Geometry check sheet. Reference: the model listing, model coordinates, mm. Face numbers are marked on the shaded views. A direction names the side the tool comes from. Give positions to 0.01 mm unless a question says otherwise; leave off trailing zeros. Loops run counter-clockwise (first coordinate to the right, second up) from the corner with the lowest first, then second, coordinate; pieces in that order, holes last. Notation, with made-up numbers: (-37.75, 47.5) -> (-33.75, 47.5) arc R13 ccw to (-33.75, 52.5) -> close; hole circle Ø3 at (38, 17). An arc over 180 degrees is marked (long way). Answer in a Markdown table with one row per item. Add a question column.
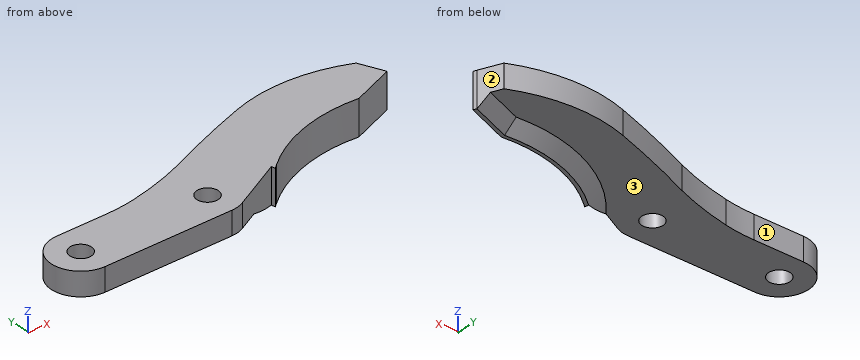
Autodesk Inventor part; units mm, degrees
ref_plane "YZ Plane" through (0, 0, 0) normal (1, 0, 0) x (0, 1, 0)
ref_plane "XZ Plane" through (0, 0, 0) normal (0, 1, 0) x (-1, 0, 0)
ref_plane "XY Plane" through (0, 0, 0) normal (0, 0, 1) x (1, 0, 0)
sketch "Náčrt1" plane through (0, 0, 0) normal (0, 0, 1) x (1, 0, 0)
  circle A0 centre (0, 0) radius 1.825
  circle A1 centre (22, 0) radius 1.825
  arc A2 (0, 5) -> (0, -5) centre (0, 0) ccw
  line L0 (0, 0) -> (-0.516, 0)
  line L1 (0, 5) -> (8.645, 5)
  arc A3 (8.645, 5) -> (13.8862, 5.4744) centre (8.645, 34.19) ccw
  arc A4 (8.645, 5) -> (8.645, 5) centre (6.8603, 48.5893) ccw
  arc A5 (58.5138, 12.7037) -> (38.8579, 13.8954) centre (47.1549, -11.9507) ccw
  line L2 (22, -5) -> (0, -5)
  line L3 (24.2622, -4.459) -> (33.0865, 0.0179)
  line L4 (22, 0) -> (22, 6.29)
  line L5 (58.5138, 12.7037) -> (60.0748, 9.0208)
  arc A6 (52.9531, 6.2627) -> (33.0865, 0.0179) centre (50.3132, -20.062) ccw
  arc A7 (22, -5) -> (24.2622, -4.459) centre (22, 0) ccw
  line L6 (52.9531, 6.2627) -> (60.0748, 9.0208)
  line L7 (23.9587, 8.3506) -> (22.7174, 7.8453)
  arc A8 (38.8579, 13.8954) -> (23.9587, 8.3506) centre (92.1034, -151.9688) ccw
  arc A9 (13.8862, 5.4744) -> (23.9587, 8.3506) centre (4.237, 58.3407) ccw
  dimension "d0" = 3.65
  dimension "d2" = 3.65
  dimension "d3" = 10
  dimension "d8" = 0.516
  dimension "d17" = 9.895
  dimension "d18" = 63.1
  dimension "d19" = 20.825
  dimension "d21" = 4
extrude "Vysunutí1" add sketch "Náčrt1" along normal blind 4 contours L1 A4 A3 A9 A8 A5 L5 L6 A6 L3 A7 L2 A2 | L1 A4 picked at (7.0586, 4.9892)
sketch "Náčrt7" plane through (0, 0, 0) normal (0, 0, -1) x (-1, 0, 0)
  arc A0 (-33.0865, 0.0179) -> (-52.9531, 6.2627) centre (-50.3132, -20.062) ccw
  line L0 (-60.0748, 9.0208) -> (-52.9531, 6.2627)
  line L1 (-60.2916, 8.4611) -> (-53.047, 5.6554)
  arc A1 (-33.8826, -0.0897) -> (-53.047, 5.6554) centre (-50.3132, -20.062) ccw
  line L2 (-33.2047, -0.6673) -> (-33.0865, 0.0179)
  line L3 (-33.8826, -0.0897) -> (-33.2047, -0.6673)
  line L4 (-59.2939, 10.8632) -> (-60.0748, 9.0208)
  line L5 (-60.2916, 8.4611) -> (-60.0748, 9.0208)
  point P0 (0, 0)
extrude "Vysunutí5" add sketch "Náčrt7" along normal blind 2 and the other way blind 4
chamfer "Zkosení3" distance 2 angle 45 2 edges at (42.3795, 5.1772, 0) (56.514, 7.6418, 0)
properties part number "lapak2" material "ABS Plastic"
1. Gauge pin test, flat ends, axial feed: pin 1 Ø3 at (y, z) = (4, 0) entering from -X; pin 2 Ø1.2 at (x, z) = (3.5, 1.5) entering from +Y. Record the tip position at first contact, or that the pin passes through.
2. Sectioned sample at B-B (x = 2.5). Enter the section's corners in (y, z).
3. Sectioned sample at A-A (z = 1.6). Count the separate pieces of the cut face and the enclosed holes in it, plus the area to 3 significant figures.
4. Material ranges on L1, parallel to Y at x = 0, z = 1.55 (3 decimals); L2, parallel to X at y = 1.25, z = 3; L3, parallel to Z at x = 13.5, y = -3.75, recorded low to high. Write a range as from..to.
5. Access from +Z, -Z, +X, -X, +Y, -Y to the whole of each face (thin tool, end or side, straight path). Record for the marked faces 1, 2 and 3.
6. Sectioned sample at D-D (z = -1.45). Enter the section's corners in (x, y), plus the area to 3 significant figures.
Response:
| question | item | result |
|---|---|---|
| 1 | pin 1 | stops at x = -4.33 |
| 1 | pin 2 | stops at y = 5 |
| 2 | outline | (-5, 0) -> (5, 0) -> (5, 4) -> (-5, 4) -> close |
| 3 | separate pieces | 1 |
| 3 | enclosed holes | 2 |
| 3 | area | 638 mm2 |
| 4 | L1 | y = -5..-1.825, 1.825..5 |
| 4 | L2 | x = -4.84..-1.33, 1.33..20.67, 23.33..35.66 |
| 4 | L3 | z = 0..4 |
| 5 | face 1 | +Z, -Z, -X, +Y |
| 5 | face 2 | +Z, -Z, +X, +Y |
| 5 | face 3 | -Z, -X, +Y |
| 6 | outline | (31.29, -0.89) -> (33.09, 0.02) -> (33.2, -0.67) -> (33.88, -0.09) arc R25.86 cw to (53.05, 5.66) -> (60.29, 8.46) -> (60.07, 9.02) -> (59.86, 9.53) -> (52.88, 6.82) arc R27.01 ccw to start |
| 6 | area | 33.9 mm2 |
